The drawing under review shows one solid part. Ordinate dimensions are in mm from its lowest x, y, z. Give positions to 0.01 mm unless a question says otherwise; leave off trailing zeros. Write each loop counter-clockwise with the first axis right and the second up, starting at its lowest first coordinate (ties: lowest second). Pieces come first, ordered by that corner, then holes.
Q1. For line 1 (Y direction, x = 4.75, z = 3) (1 decimal); line 2 (X direction, y = 12.25, z = 2) (1 decimal); line 3 (X direction, y = 7, z = 5.25) (1 decimal), list the stretches that pass through material, from the lowest coordinate up.
Q2. We need section C-C (z = 3.5). Write out the cut boundary in (x, y) (1 decimal).
Q3. We need section A-A (z = 6). Write out the cut boundary in (x, y) (1 decimal).
Q4. Mouldability with a two-part tool opening along Z and no side actions: class the marked faces 1, 2 and 3 as released by +Z, released by -Z, zero draft, split by the parting line, or undercut.
Q5. We need section B-B (y = 9.25). Give the number of separate pieces and of enclosed holes in the cut face, then the cut area to 3 significant figures.
Q6. Insertion check: P1, Ø1.5, axis at y = 9.5, z = 2.5, coming from the -X side; P2, Ø2, axis at y = 13, z = 1.5, coming from the -X side; P3, Ø3, axis at x = 11, z = 4.5, coming from the +Y side. Each pin has a flat end and moves straight along its axis. Give the tip position at first contact, or say it passes through.
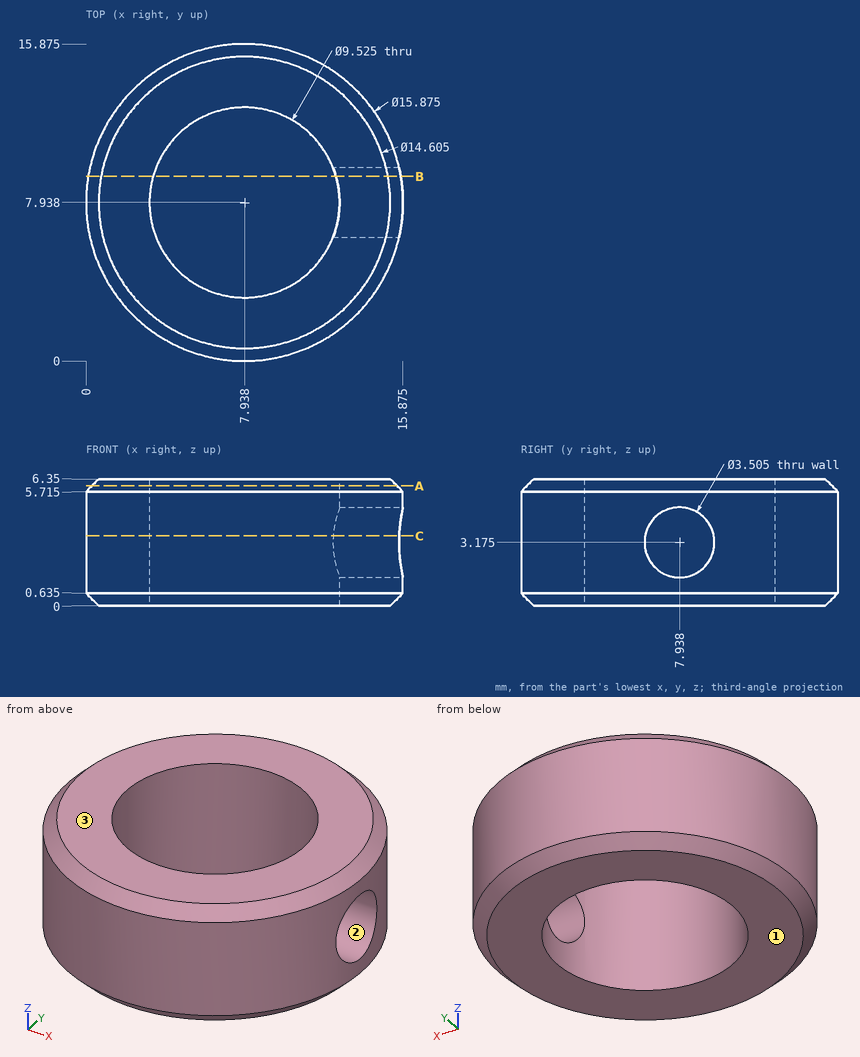
Computed:
1. line 1: y = 0.7 to 4.4, 11.5 to 15.2
1. line 2: x = 1.3 to 5.9, 10 to 14.6
1. line 3: x = 0.1 to 3.3, 12.6 to 15.8
2. outline: (12.4, 6.2) arc R4.8 cw (long way) to (12.4, 9.7) - (15.7, 9.7) arc R7.9 ccw (long way) to (15.7, 6.2) - close
3. outline: circle Ø15.3 at (7.9, 7.9); hole circle Ø9.5 at (7.9, 7.9)
4. face 1: released by -Z
4. face 2: undercut
4. face 3: released by +Z
5. separate pieces: 3
5. enclosed holes: 0
5. area: 32.9 mm2
6. P1: stops at x = 0.04
6. P2: stops at x = 1.12
6. P3: stops at y = 15.72
